CAD build for the part. Positions are in the model's coordinates, mm. A direction names the side the tool comes from. Coordinates: 2 decimals unless noted, no trailing zeros. Loops run counter-clockwise (first coordinate to the right, second up) from the corner with the lowest first, then second, coordinate; pieces in that order, holes last. Notation, with made-up numbers: (13, 43) -> (62, 43) arc R21 cw to (62, 71) -> close; hole circle Ø11 at (57.5, 86.25). An arc over 180 degrees is marked (long way). Write each question's results on one line, items separated by ' | '.
from build123d import *

# Parameters (mm, degrees)
F1_DEPTH = 19.05
F2_W     = 469.9
F2_H     = 19.05
F3_DEPTH = 15.875


with BuildPart() as f1:
    # F0 (on Right) → F1 (new body)
    with BuildSketch(Plane.YZ):
        Polygon((-599.02876, -133.371351), (-618.07876, -133.371351), (-618.07876, -174.011351), (-599.02876, -174.011351), (-599.02876, -214.651351), (-618.07876, -214.651351), (-618.07876, -255.291351), (-599.02876, -255.291351), (-599.02876, -295.931351), (-618.07876, -295.931351), (-618.07876, -335.618851), (-599.02876, -335.618851), (-129.12876, -335.618851), (-110.07876, -335.618851), (-110.07876, -295.931351), (-129.12876, -295.931351), (-129.12876, -255.291351), (-110.07876, -255.291351), (-110.07876, -214.651351), (-129.12876, -214.651351), (-129.12876, -174.011351), (-110.07876, -174.011351), (-110.07876, -133.371351), (-129.12876, -133.371351), (-129.12876, -92.731351), (-599.02876, -92.731351), align=None)
    extrude(amount=F1_DEPTH)

    # F2 (on face) → F3 (cut)
    with BuildSketch(Plane.YZ.offset(19.05)):
        with Locations((-364.07876, -102.256351)):
            Rectangle(F2_W, F2_H)
    extrude(amount=-F3_DEPTH, mode=Mode.SUBTRACT)


solid = f1.part
1) Which spindle directions (+Z, -Z, +X, -X, +Y, -Y) get a long thin tool onto all of the face, cutting with end or side? Do faces 5 (the flat face through (9, -599.029, -194)), 6 (the flat face through (9, -129.129, -195)), 7 (the flat face through (7, -129.129, -118)). Say none if no direction does.
Outcome:
face 5: +X, -X, -Y | face 6: +X, -X, +Y | face 7: +Z, +X, -X, +Y
2) Pin check, flat tips, straight feed: pin 1 (5.5 mm diameter, centred on x = 14.5, y = -610, fed in from +Z); pin 2 (5 mm diameter, centred on x = 6.5, y = -252.5, fed in from +Z); pin 3 (9.5 mm diameter, centred on y = -314, z = -99.5, fed in from +X) (3 decimals). Stop position of each tip, or through.
Outcome:
pin 1: stops at z = -133.37 | pin 2: stops at z = -111.78 | pin 3: stops at x = 3.175
3) Slice it at A-A (x = 8.25). Write the cut outline in (y, z), then the cut area to 3 significant figures.
Outcome:
outline: (-618.08, -335.62) -> (-110.08, -335.62) -> (-110.08, -295.93) -> (-129.13, -295.93) -> (-129.13, -255.29) -> (-110.08, -255.29) -> (-110.08, -214.65) -> (-129.13, -214.65) -> (-129.13, -174.01) -> (-110.08, -174.01) -> (-110.08, -133.37) -> (-129.13, -133.37) -> (-129.13, -111.78) -> (-599.03, -111.78) -> (-599.03, -133.37) -> (-618.08, -133.37) -> (-618.08, -174.01) -> (-599.03, -174.01) -> (-599.03, -214.65) -> (-618.08, -214.65) -> (-618.08, -255.29) -> (-599.03, -255.29) -> (-599.03, -295.93) -> (-618.08, -295.93) -> close | area: 110,000 mm^2
4) Slice it at C-C (z = -202.5). Write the cut outline in (x, y), then the cut area to 3 significant figures.
Outcome:
outline: (0, -599.03) -> (19.05, -599.03) -> (19.05, -129.13) -> (0, -129.13) -> close | area: 8,950 mm^2
5) Drill centre lines: L1, parallel to Z at x = 16, y = -195.5; L2, parallel to Y at x = 8, z = -256.5; L3, parallel to X at y = -483, z = -107 (3 decimals). Where is each one in solid material? Low to high. Write a range as from..to.
Outcome:
L1: z = -335.62..-111.78 | L2: y = -599.03..-129.13 | L3: x = 0..3.175
6) Two-plate mould, pull along Z, no slides. Class faces 1 (the flat face through (9, -608, -133.371)), 2 (the flat face through (9, -368, -335.619)), 3 (the flat face through (9, -129.129, -276)), 4 (the flat face through (7, -599.029, -117)): pulls with the +Z half, pulls with the -Z half, needs draft (parallel to the pull), parting line crosses it, or undercut.
Outcome:
face 1: pulls with the +Z half | face 2: pulls with the -Z half | face 3: undercut | face 4: needs draft
7) Slice it at B-B (y = -249.5). Write the cut outline in (x, z) (3 decimals).
Outcome:
outline: (0, -335.619) -> (19.05, -335.619) -> (19.05, -111.781) -> (3.175, -111.781) -> (3.175, -92.731) -> (0, -92.731) -> close
